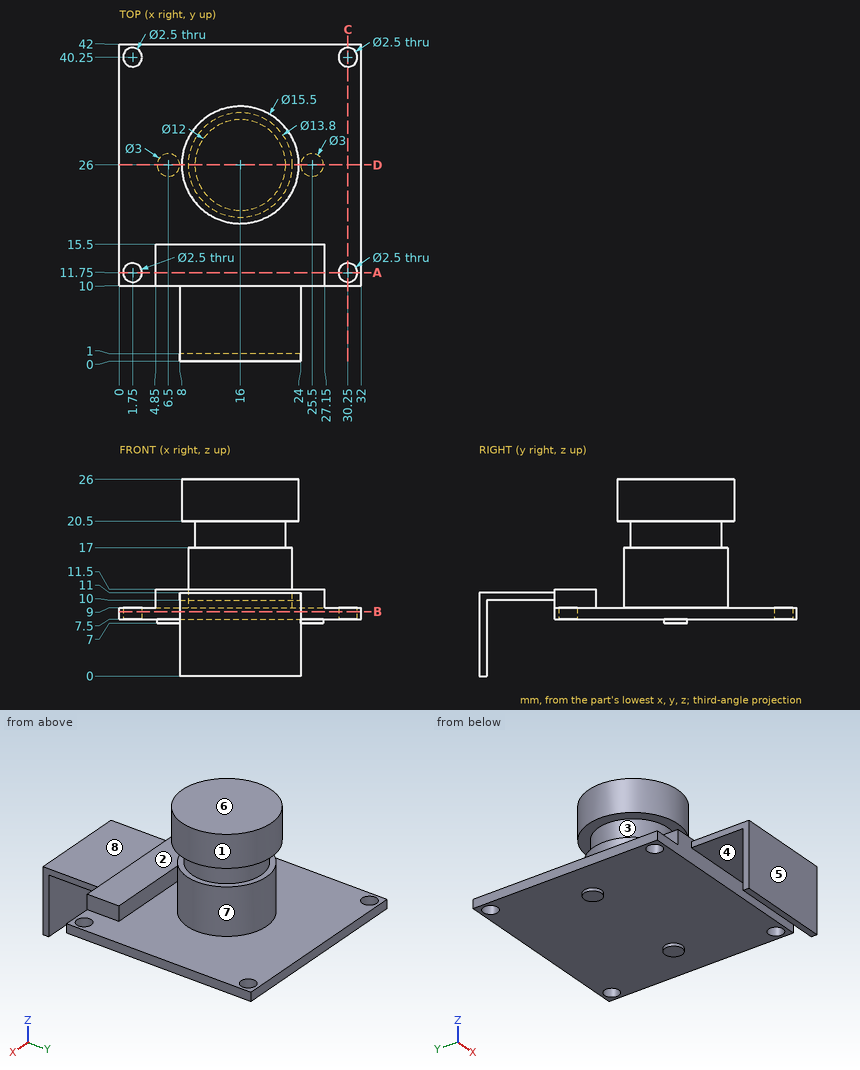
Here's the drawing with two shaded views (mm, measured from the low corner). I have some questions. A direction names the side the tool comes from. Round coordinates to 2 decimals unless told otherwise and drop trailing zeros. Loops run counter-clockwise (first coordinate to the right, second up) from the corner with the lowest first, then second, coordinate; pieces in that order, holes last. Notation, with made-up numbers: (-20.75, -25) - (36.25, -25) arc R27 ccw to (36.25, 3) - close; hole circle Ø6 at (37, -6.5). An arc over 180 degrees is marked (long way). Use CSV: the item, a comma, the result in double quotes. Start each with the question number.
1) If we section it at B-B on z = 8.5: Write out the boundary of the cut face in (x, y), plus the area to 3 significant figures.
2) If we section it at D-D on y = 26: Write out the boundary of the cut face in (x, z).
3) We'd pull the mould along Z, two halves only. Please class the marked faces 1, 2 and 3: released by +Z, released by -Z, zero draft, split by the parting line, or undercut.
4) For the marked faces 4, 5, 6, 7 and 8, which set-ups out of +Z, -Z, +X, -X, +Y, -Y let a thin tool reach every point of the face, with its end or its side?
5) If we section it at A-A on y = 11.75: Write out the boundary of the cut face in (x, z), plus the area to 4 significant figures.
6) For pin 1 Ø3 at (x, y) = (8, 24) entering from -Z; pin 2 Ø3 at (x, y) = (1.75, 11.75) entering from -Z; pin 3 Ø1.6 at (x, y) = (21, 13) entering from +Z, each with a flat end and sliding along its axis, tell me the tip position at first contact or that it passes through.
7) Please list where these lines run through material, in increasing order: probe 1 along Y at (x, z) = (30.25, 8.35); probe 2 along Z at (x, y) = (12.5, 20); probe 3 along Z at (x, y) = (12.5, 2.5). Write a range as [from, to].
8) If we section it at C-C on x = 30.25: Write out the boundary of the cut face in (y, z).
Geometry results:
1,outline,"(0, 10) - (32, 10) - (32, 42) - (0, 42) - close; (8, 0) - (24, 0) - (24, 1) - (8, 1) - close; hole circle Ø2.5 at (1.75, 11.75); hole circle Ø2.5 at (1.75, 40.25); hole circle Ø2.5 at (30.25, 11.75); hole circle Ø2.5 at (30.25, 40.25)"
1,area,"1,020 mm2"
2,outline,"(0, 7.5) - (5, 7.5) - (5, 7) - (8, 7) - (8, 7.5) - (24, 7.5) - (24, 7) - (27, 7) - (27, 7.5) - (32, 7.5) - (32, 9) - (22.9, 9) - (22.9, 17) - (22, 17) - (22, 20.5) - (23.75, 20.5) - (23.75, 26) - (8.25, 26) - (8.25, 20.5) - (10, 20.5) - (10, 17) - (9.1, 17) - (9.1, 9) - (0, 9) - close"
3,face 1,"zero draft"
3,face 2,"released by +Z"
3,face 3,"undercut"
4,face 4,"-Z, +X, -X"
4,face 5,"+Z, -Z, +X, -X, -Y"
4,face 6,"+Z, +X, -X, +Y, -Y"
4,face 7,"none"
4,face 8,"+Z, +X, -X, -Y"
5,outline,"(0, 7.5) - (0.5, 7.5) - (0.5, 9) - (0, 9) - close; (3, 7.5) - (29, 7.5) - (29, 9) - (27.15, 9) - (27.15, 11.5) - (4.85, 11.5) - (4.85, 9) - (3, 9) - close; (31.5, 7.5) - (32, 7.5) - (32, 9) - (31.5, 9) - close"
5,area,"96.25 mm2"
6,pin 1,"stops at z = 7"
6,pin 2,"stops at z = 7.5"
6,pin 3,"stops at z = 11.5"
7,probe 1,"y = [10, 10.5], [13, 39], [41.5, 42]"
7,probe 2,"z = [7.5, 9], [20.5, 26]"
7,probe 3,"z = [10, 11]"
8,outline,"(10, 7.5) - (10.5, 7.5) - (10.5, 9) - (10, 9) - close; (13, 7.5) - (39, 7.5) - (39, 9) - (13, 9) - close; (41.5, 7.5) - (42, 7.5) - (42, 9) - (41.5, 9) - close"
